Input: part model. Units: mm. Frame: model coordinates. Face numbers are marked on the shaded views. A direction names the side the tool comes from. Give positions to 0.01 mm unless a question says otherwise; leave off trailing zeros. Write each loop counter-clockwise with the first axis right and the second up, starting at its lowest first coordinate (ties: lowest second). Pieces come first, ordered by that corner, then holes. Notation, with made-up numbers: (-19, 27.25) -> (36, 27.25) arc R17 ccw to (36, 46.25) -> close; hole circle Ø6 at (-17, -23). An arc over 180 degrees is marked (long way). Return JSON: item names as keys, results as strings. Group by question number.
Item 1: Set-up query: the marked faces 1, 2 and 3. Return all of +Z, -Z, +X, -X, +Y, -Y with unobstructed straight access to the full face (end or side cutting, diameter ignored); none if empty.
Item 2: Pin query (flat end, axial travel): P1, Ø2, axis at x = 15, y = 1, coming from the +Z side. Return the tip coordinate at first contact, or that it passes through.
Item 3: Section A-A, the plane z = 23.75. Return loops of the section in (x, y).
Item 4: Section C-C, the plane x = -10.5. Return loops of the section in (y, z).
Item 5: Mould query, pull axis Y, two halves, no side actions, for the marked faces 4, 5 and 6. Classes: released by +Y, released by -Y, zero draft, split by the parting line, or undercut.
Item 6: Section D-D, the plane y = -21.5. Return loops of the section in (x, z).
Item 7: Line query: line 1 (X direction, y = 0, z = 15); line 2 (Y direction, x = -35, z = 8.75); line 3 (X direction, y = 4, z = 14.75). Output: solid intervals per line, ascending. Write a range as [from, to].
Item 8: Section B-B, the plane y = 7. Return loops of the section in (x, z), then the cut area to 3 significant figures.
from build123d import *

# Parameters (mm, degrees)
F0_W     = 80
F0_H     = 80
F1_DEPTH = 25
F2_R     = 34
F3_DEPTH = 20
F4_R     = 9
F5_DEPTH = 20
F7_DEPTH = 20
F8_W     = 6
F8_H     = 16
F9_DEPTH = 20


with BuildPart() as f1:
    # F0 (on Top) → F1 (new body)
    with BuildSketch(Plane.XY):
        Rectangle(F0_W, F0_H)
    extrude(amount=F1_DEPTH)

    # F2 (on face) → F3 (cut)
    with BuildSketch(Plane.XY.offset(25)):
        Circle(F2_R)
    extrude(amount=-F3_DEPTH, mode=Mode.SUBTRACT)

    # F4 (on face) → F5 (join)
    with BuildSketch(Plane.XY.offset(5)):
        Circle(F4_R)
    extrude(amount=F5_DEPTH)

    # F6 (on face) → F7 (cut, through all)
    with BuildSketch(Plane.XY.offset(25)):
        with BuildLine():
            Line((-34, 34), (-34, 0))
            Line((-34, 0), (-9, 0))
            ThreePointArc((-9, 0), (-6.363961, 6.363961), (0, 9))
            Line((0, 9), (0, 34))
            Line((0, 34), (-34, 34))
        make_face()
    extrude(amount=-F7_DEPTH, mode=Mode.SUBTRACT)

    # F8 (on face) → F9 (cut, through all)
    with BuildSketch(Plane.XY.offset(25)):
        with Locations((-37, 26)):
            Rectangle(F8_W, F8_H)
    extrude(amount=-F9_DEPTH, mode=Mode.SUBTRACT)


solid = f1.part
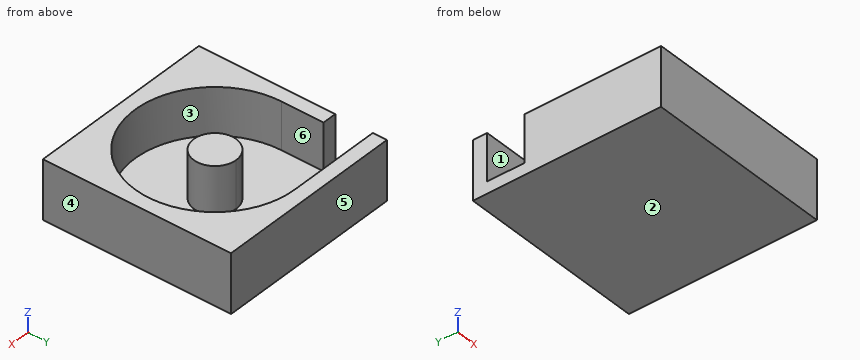
Answer below:
{
 "1": {"face 1": "+Z, -X", "face 2": "-Z, +X, -X, +Y, -Y", "face 3": "+Z"},
 "2": {"P1": "stops at z = 5"},
 "3": {"outline": "(-40, -40) -> (40, -40) -> (40, 40) -> (-40, 40) -> (-40, 34) -> (0, 34) arc R34 cw (long way) to (-34, 0) -> (-34, 18) -> (-40, 18) -> close; circle Ø18 at (0, 0)"},
 "4": {"outline": "(-40, 0) -> (40, 0) -> (40, 25) -> (34, 25) -> (34, 5) -> (-32.34, 5) -> (-32.34, 25) -> (-40, 25) -> close"},
 "5": {"face 4": "zero draft", "face 5": "released by +Y", "face 6": "undercut"},
 "6": {"outline": "(-40, 0) -> (40, 0) -> (40, 25) -> (26.34, 25) -> (26.34, 5) -> (-26.34, 5) -> (-26.34, 25) -> (-40, 25) -> close"},
 "7": {"line 1": "x = [-40, -34], [-9, 9], [34, 40]", "line 2": "y = [-40, 18], [34, 40]", "line 3": "x = [-40, -34], [-8.06, 8.06], [33.76, 40]"},
 "8": {"outline": "(-40, 0) -> (40, 0) -> (40, 25) -> (33.27, 25) -> (33.27, 5) -> (5.66, 5) -> (5.66, 25) -> (-5.66, 25) -> (-5.66, 5) -> (-34, 5) -> (-34, 25) -> (-40, 25) -> close", "area": "881 mm2"}
}
